from build123d import *

# Parameters (mm, degrees)
SCHIZZO1_W                   = 8.27
SCHIZZO1_H                   = 12
ESTRUSIONE_ESTRUSIONE1_DEPTH = 4
RACCORDO1_R                  = 2
RACCORDO2_R                  = 2
SCHIZZO3_R                   = 1.62
TAGLIO_ESTRUSIONE1_DEPTH     = 4
SCHIZZO4_R                   = 2.5
ESTRUSIONE_ESTRUSIONE2_DEPTH = 12
SCHIZZO5_R                   = 2.5
ESTRUSIONE_ESTRUSIONE3_DEPTH = 25


with BuildPart() as part:
    # Schizzo1 → Estrusione-Estrusione1 (new body)
    with BuildSketch(Plane.XY):
        Rectangle(SCHIZZO1_W, SCHIZZO1_H)
    extrude(amount=ESTRUSIONE_ESTRUSIONE1_DEPTH)

    # Raccordo1
    raccordo1_edges = [part.edges().sort_by_distance(p)[0] for p in [
        (4.135, 6, 2),
    ]]
    fillet(raccordo1_edges, radius=RACCORDO1_R)

    # Raccordo2
    raccordo2_edges = [part.edges().sort_by_distance(p)[0] for p in [
        (4.135, -6, 2),
        (-4.135, -6, 2),
        (-4.135, 6, 2),
    ]]
    fillet(raccordo2_edges, radius=RACCORDO2_R)

    # Schizzo3 → Taglio-Estrusione1 (cut)
    with BuildSketch(Plane.XY.offset(4)):
        with Locations((0, 3.5)):
            Circle(SCHIZZO3_R)
    extrude(amount=-TAGLIO_ESTRUSIONE1_DEPTH, mode=Mode.SUBTRACT)

    # Schizzo4 → Estrusione-Estrusione2 (add)
    with BuildSketch(Plane.XY.offset(4)):
        with Locations((0, -1.86312089)):
            Circle(SCHIZZO4_R)
    extrude(amount=ESTRUSIONE_ESTRUSIONE2_DEPTH)

    # Schizzo5 → Estrusione-Estrusione3 (add)
    with BuildSketch(Plane(origin=(0, 0.6, 0), x_dir=(1, 0, 0), z_dir=(0, 1, 0))):
        with Locations(Location((0, -13.4915802, 0), (0, 0, 270))):
            Circle(SCHIZZO5_R)
    extrude(amount=-ESTRUSIONE_ESTRUSIONE3_DEPTH)


solid = part.part
Can you work these out from the model? Positions are in its coordinate system, mm. A direction names the side the tool comes from. Coordinates: 2 decimals unless noted, no trailing zeros. Order: outer loops, then holes, each group sorted by start corner. A loop starts at its lowest first (then second) coordinate and runs counter-clockwise, first axis right, second up. Notation, with made-up numbers: M -4.75,-26 L 7.25,-26 A32 ccw 7.25,9 Z; hole C 13,69.25 d3. An arc over 180 degrees is marked long. Write item = value, one per line.
(1) Suppose I cut it at D-D on y = -2.5. Please give me the cut outline in (x, z) (3 decimals).
Results are:
outline = M -4.135,0 L 4.135,0 L 4.135,4 L 2.418,4 L 2.418,12.855 A2.5 ccw 2.418,14.128 L 2.418,16 L -2.418,16 L -2.418,14.128 A2.5 ccw -2.418,12.855 L -2.418,4 L -4.135,4 Z
(2) Suppose I cut it at A-A on y = 3.5. Please give me the cut outline in (x, z) (3 decimals), plus the area to 3 significant figures.
Results are:
outline = M -4.135,0 L -1.62,0 L -1.62,4 L -4.135,4 Z; M 1.62,0 L 4.135,0 L 4.135,4 L 1.62,4 Z
area = 20.1 mm2
(3) For faces 1 (the face through (-0.325, 0.616, 8.583)), 2 (the face through (-2.5, -0.1, 13.4)), 3 (the face through (1, 0.6, 13)), 4 (the face through (0, -6, 2)), 5 (the face through (2.5, -0.1, 13.5)), which set-ups out of +Z, -Z, +X, -X, +Y, -Y let a thin tool reach every point of the face, with its end or its side?
Results are:
face_1 = none
face_2 = -X, +Y
face_3 = +Z, +X, +Y
face_4 = -Z, +X, -X, -Y
face_5 = +X, +Y
(4) Suppose I cut it at C-C on z = 6. Please give me the cut outline in (x, y).
Results are:
outline = C 0,-1.86 d5
(5) I need wall thicknesses on line 1 along Y through (x, z) = (0, 1.1); line 2 along Y through (x, z) = (0, 11.25); line 3 along Z through (x, y) = (3.25, 1.5). Which ranges of each line are inside material? Lowest first, please. Write a range as [from, to].
Results are:
line_1 = [-6, 1.88], [5.12, 6]
line_2 = [-24.4, 0.64]
line_3 = [0, 4]
(6) For pin 1 Ø1 at (y, z) = (-6, 2.5) entering from +X; pin 2 Ø3 at (x, z) = (-1, 9.5) entering from +Y; pin 3 Ø5 at (y, z) = (-18.5, 14.5) entering from -X, each with a flat end and sliding along its axis, tell me the tip position at first contact or that it passes through.
Results are:
pin_1 = 3.46
pin_2 = 0.64
pin_3 = -2.5
